from build123d import *

# Parameters (mm, degrees)
ESBO_O1_R                = 4
ESBO_O1_R_2              = 2
RESSALTO_EXTRUS_O1_DEPTH = 19
FILETE1_R                = 7
ESBO_O3_R                = 5.497341607
CORTE_EXTRUS_O1_DEPTH    = 12.5
CORTE_EXTRUS_O5_DEPTH    = 33.95451427


with BuildPart() as part:
    # Esboço1 → Ressalto-extrusão1 (new body)
    with BuildSketch(Plane.XY):
        with BuildLine():
            Line((5, -9.5), (5, 0))
            Line((5, 0), (5, 9.5))
            Line((5, 9.5), (-11.877501001, 9.5))
            ThreePointArc((-11.877501001, 9.5), (-25, 0), (-11.877501001, -9.5))
            Line((-11.877501001, -9.5), (5, -9.5))
        make_face()
        with Locations((-15, 0)):
            Circle(ESBO_O1_R, mode=Mode.SUBTRACT)
        Circle(ESBO_O1_R_2, mode=Mode.SUBTRACT)
    extrude(amount=RESSALTO_EXTRUS_O1_DEPTH)

    # Filete1
    filete1_edges = [part.edges().sort_by_distance(p)[0] for p in [
        (-3.4387505, 9.5, 0),
        (-3.4387505, 9.5, 19),
        (-3.4387505, -9.5, 19),
        (-3.4387505, -9.5, 0),
    ]]
    fillet(filete1_edges, radius=FILETE1_R)

    # Esboço3 → Corte-extrusão1 (cut)
    with BuildSketch(Plane(origin=(5, 0, 0), x_dir=(0, 0, -1), z_dir=(1, 0, 0))):
        with Locations(Location((-9.5, 0, 0), (0, 0, 90))):
            Circle(ESBO_O3_R)
    extrude(amount=-CORTE_EXTRUS_O1_DEPTH, mode=Mode.SUBTRACT)

    # Esboço5 → Corte-extrusão5 (cut, through all)
    with BuildSketch(Plane(origin=(0, 0, 0), x_dir=(-1, 0, 0), z_dir=(0, 0, -1))):
        with BuildLine():
            Line((9.035898385, 0), (9.035898385, -2))
            Line((9.035898385, -2), (11.535898385, -2))
            ThreePointArc((11.535898385, -2), (11, 0), (11.535898385, 2))
            Line((11.535898385, 2), (9.035898385, 2))
            Line((9.035898385, 2), (9.035898385, 0))
        make_face()
    extrude(amount=-CORTE_EXTRUS_O5_DEPTH, mode=Mode.SUBTRACT)


solid = part.part
The listing builds one solid part. Answer for the finished solid, in the listing's coordinates (mm). A direction names the side the tool comes from. Round coordinates to 2 decimals unless told otherwise and drop trailing zeros. Loops run counter-clockwise (first coordinate to the right, second up) from the corner with the lowest first, then second, coordinate; pieces in that order, holes last. Notation, with made-up numbers: M 13,4 L 23,4 A24 cw 23,42 Z; hole C -33,12.5 d10. An arc over 180 degrees is marked long. Return JSON: item names as keys, results as strings.
Q1. The mould has two halves that part along X. Classify faces 5 (the face through (-10, -2, 9)), 6 (the face through (-4, -9.5, 9)), 7 (the face through (-7.5, 0, 10)): released by +X, released by -X, zero draft, split by the parting line, or undercut.
Results list:
{"face 5": "undercut", "face 6": "zero draft", "face 7": "released by +X"}
Q2. Each of these flat-tipped pins is pushed along its axis until it touches: pin 1 Ø10 at (x, z) = (-3, 10) entering from +Y; pin 2 Ø2 at (x, z) = (0.5, 15.5) entering from +Y; pin 3 Ø6 at (y, z) = (-6.5, 2) entering from -X. Where does it stop, or does it pass through?
Results list:
{"pin 1": "stops at y = 9.5", "pin 2": "stops at y = 9.04", "pin 3": "stops at x = -24.37"}
Q3. Find section B-B, the plane x = 3. Determine the outline of the cut face in (y, z).
Results list:
{"outline": "M -9.5,7 A7 ccw -2.5,0 L 2.5,0 A7 ccw 9.5,7 L 9.5,12 A7 ccw 2.5,19 L -2.5,19 A7 ccw -9.5,12 Z; hole C 0,9.5 d10.99"}
Q4. Which of the six approach directions +Z, -Z, +X, -X, +Y, -Y give full straight-line access (tool end or side, diameter ignored) to faces 1 (the face through (-10, 2, 9)), 2 (the face through (-1.7, 7.5, 2.1)), 3 (the face through (-1.4, -7.5, 2.1)), 4 (the face through (-3, 9.5, 9))?
Results list:
{"face 1": "+Z, -Z", "face 2": "-Z, +X, +Y", "face 3": "-Z, +X, -Y", "face 4": "+Z, -Z, +X, +Y"}
Q5. Find section D-D, the plane z = 1.25. Determine the outline of the cut face in (x, y).
Results list:
{"outline": "M -7.39,-6.49 L 5,-6.49 L 5,6.49 L -7.39,6.49 A10 ccw long Z; hole M -11.54,-2 L -9.04,-2 L -9.04,2 L -11.54,2 A4 ccw long Z; hole C 0,0 d4"}
Q6. Find section C-C, the plane z = 9.5. Determine the outline of the cut face in (x, y), plus the area to 3 significant figures.
Results list:
{"outline": "M -11.88,-9.5 L 5,-9.5 L 5,-5.5 L -7.5,-5.5 L -7.5,5.5 L 5,5.5 L 5,9.5 L -11.88,9.5 A10 ccw long Z; hole M -11.54,-2 L -9.04,-2 L -9.04,2 L -11.54,2 A4 ccw long Z", "area": "343 mm2"}
Q7. Find section A-A, the plane y = 0. Determine the outline of the cut face in (x, z).
Results list:
{"outline": "M -25,0 L -19,0 L -19,19 L -25,19 Z; M -9.04,0 L -2,0 L -2,4 L -7.5,4 L -7.5,15 L -2,15 L -2,19 L -9.04,19 Z; M 2,0 L 5,0 L 5,4 L 2,4 Z; M 2,15 L 5,15 L 5,19 L 2,19 Z"}
Q8. Find the intervals of material crossed by line 1 along X through (y, z) = (0, 1.3); line 2 along Y through (x, z) = (-15, 5.5); line 3 along X through (y, z) = (0, 14.5), in increasing order. Write a range as from..to.
Results list:
{"line 1": "x = -25..-19, -9.04..-2, 2..5", "line 2": "y = -10..-4, 4..10", "line 3": "x = -25..-19, -9.04..-7.5"}
